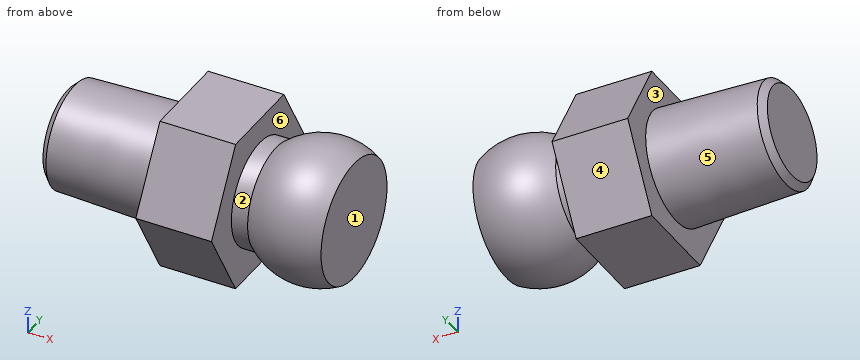
from build123d import *

# Parameters (mm, degrees)
SKETCH_2_R          = 14
CUT_EXTRUDE_1_DEPTH = 6.9


with BuildPart() as part:
    # Sketch 1 → Revolve 1 (revolve)
    with BuildSketch(Plane.XY, mode=Mode.PRIVATE) as revolve_1_sk:
        with BuildLine():
            Line((0, 0), (0, 4.158121832))
            Line((0, 4.158121832), (0.59972308, 4.757844912))
            Line((0.59972308, 4.757844912), (10.6, 5.070048976))
            Line((10.6, 5.070048976), (10.6, 12))
            Line((10.6, 12), (17.5, 12))
            Line((17.5, 12), (17.5, 4.75))
            Line((17.5, 4.75), (18.982041495, 4.75))
            ThreePointArc((18.982041495, 4.75), (22.419985488, 6.249612989), (26.1, 5.524498371))
            Line((26.1, 5.524498371), (26.1, 0))
            Line((26.1, 0), (0, 0))
        make_face()
    revolve(revolve_1_sk.sketch.rotate(Axis((26.1, 0, 0), (-1, 0, 0)), 270), axis=Axis((26.1, 0, 0), (-1, 0, 0)))

    # Sketch 2 → Cut-Extrude 1 (cut)
    with BuildSketch(Plane.ZY.offset(-10.6)):
        Circle(SKETCH_2_R)
        Polygon((0, -8.082903769), (7, -4.041451884), (7, 4.041451884), (0, 8.082903769), (-7, 4.041451884), (-7, -4.041451884), align=None, mode=Mode.SUBTRACT)
    extrude(amount=-CUT_EXTRUDE_1_DEPTH, mode=Mode.SUBTRACT)


solid = part.part
Design review of the part built by this model. Coordinates are the model's own, in mm. Face numbers are marked on the shaded views. A direction names the side the tool comes from. Coordinates: 2 decimals unless noted, no trailing zeros. Order: outer loops, then holes, each group sorted by start corner. A loop starts at its lowest first (then second) coordinate and runs counter-clockwise, first axis right, second up.
Item 1: For line 1 (X direction, y = -6.5, z = -2); line 2 (Z direction, x = 16, y = 5.75); line 3 (X direction, y = -5, z = 1), list the stretches that pass through material, from the lowest coordinate up.
Item 2: Take a section at B-B, the plane x = 12.25. Write out the cut boundary in (y, z), then the cut area to 3 significant figures.
Item 3: The part is to be moulded in two halves that separate along X. For the marked faces 1, 2 and 3, say which applies: pulls with the +X half, pulls with the -X half, needs draft (parallel to the pull), parting line crosses it, or undercut.
Item 4: Take a section at A-A, the plane y = 0. Write out the cut boundary in (x, z).
Item 5: Take a section at C-C, the plane y = -7. Write out the cut boundary in (x, z), then the cut area to 3 significant figures.
Item 6: For pin 1 Ø1 at (x, z) = (14, -4) entering from +Y; pin 2 Ø1 at (x, z) = (8.5, -4) entering from +Y; pin 3 Ø6 at (x, z) = (6, 2) entering from +Y, all flat-tipped, find the tip position at first contact; note any pin that passes through.
Item 7: For the marked faces 4, 5 and 6, list the 3-axis set-ups (+Z, -Z, +X, -X, +Y, -Y) from which the entire face can be reached by the end or side of a thin tool; tool diameter is ignored.
The answers:
1. line 1: x = 10.6 to 17.5
1. line 2: z = -4.04 to 4.04
1. line 3: x = 10.6 to 17.5, 19.42 to 26.1
2. outline: (-8.08, 0) - (-4.04, -7) - (4.04, -7) - (8.08, 0) - (4.04, 7) - (-4.04, 7) - close
2. area: 170 mm2
3. face 1: pulls with the +X half
3. face 2: undercut
3. face 3: pulls with the -X half
4. outline: (0, -4.16) - (0.6, -4.76) - (10.6, -5.07) - (10.6, -7) - (17.5, -7) - (17.5, -4.75) - (18.98, -4.75) arc R6.29 ccw to (26.1, -5.52) - (26.1, 5.52) arc R6.29 ccw to (18.98, 4.75) - (17.5, 4.75) - (17.5, 7) - (10.6, 7) - (10.6, 5.07) - (0.6, 4.76) - (0, 4.16) - close
5. outline: (10.6, -1.88) - (17.5, -1.88) - (17.5, 1.88) - (10.6, 1.88) - close
5. area: 25.9 mm2
6. pin 1: stops at y = 6.06
6. pin 2: stops at y = 3.58
6. pin 3: stops at y = 5
7. face 4: -Z, +X, -X, +Y
7. face 5: -X
7. face 6: none
